CAD build for the part. Positions are in the model's coordinates, mm. A direction names the side the tool comes from. Round coordinates to 2 decimals unless told otherwise and drop trailing zeros. Loops run counter-clockwise (first coordinate to the right, second up) from the corner with the lowest first, then second, coordinate; pieces in that order, holes last. Notation, with made-up numbers: M 26,83 L 74,83 A20 ccw 74,122 Z; hole C -29.5,-24.5 d3. An arc over 180 degrees is marked long. Use a Markdown table: item, result. Add a question column.
(1) Band-saw the part on D-D, the plane y = -10.5. Write the cut outline in (x, z), and give its area (3 significant figures).
(2) Flat gauge pins, fed straight in: P1, Ø8, axis at x = 13.5, y = 5, coming from the +Z side; P2, Ø2, axis at y = -2, z = 27, coming from the +X side; P3, Ø1, axis at y = -4, z = 107, coming from the -X side; P4, Ø5, axis at x = 16.5, z = 101, coming from the -Y side. Where does each tip first touch, or does it go through?
(3) Which spindle directions (+Z, -Z, +X, -X, +Y, -Y) get a long thin tool onto all of the face, cutting with end or side? Do faces 1 (the face through (13.9, 0, 54)), 2 (the face through (-13.9, 0, 54)), 3 (the face through (0.42, -0.78, 135.95)). Say none if no direction does.
(4) Wall check: L1, parallel to Z at x = 7.5, y = 9; L2, parallel to X at y = -3.25, z = 33.5; L3, parallel to Y at x = -10.5, z = 129.5. Give the ranges that are in metal, low to high.
(5) Band-saw the part on A-A, the plane x = 0. Write the cut outline in (y, z), and give its area (3 significant figures).
(6) Band-saw the part on C-C, the plane z = 66.5. Write the cut outline in (x, y), and give its area (3 significant figures).
(7) Band-saw the part on B-B, the plane y = 0. Write the cut outline in (x, z).
from build123d import *

# Parameters (mm, degrees)
F0_W     = 27.8
F0_H     = 27.8
F1_DEPTH = 110
F2_R     = 6
F3_DEPTH = 20
F4_R     = 6
F5_DEPTH = 30


with BuildPart() as f1:
    # F0 (on Top) → F1 (new body)
    with BuildSketch(Plane.XY):
        Rectangle(F0_W, F0_H)
    extrude(amount=F1_DEPTH)

    # F2 (on face) → F3 (join)
    with BuildSketch(Plane.XY.offset(110)):
        Circle(F2_R)
    extrude(amount=F3_DEPTH)

    # F4 (on Right) → F5 (join, symmetric)
    with BuildSketch(Plane.YZ):
        with Locations((0, 130)):
            Circle(F4_R)
    extrude(amount=F5_DEPTH, both=True)


solid = f1.part
Return value:
| question | item | result |
|---|---|---|
| 1 | outline | M -13.9,0 L 13.9,0 L 13.9,110 L -13.9,110 Z |
| 1 | area | 3,060 mm^2 |
| 2 | P1 | z = 135.92 |
| 2 | P2 | x = 13.9 |
| 2 | P3 | x = -13.9 |
| 2 | P4 | through |
| 3 | face 1 | -Z, +X, +Y, -Y |
| 3 | face 2 | -Z, -X, +Y, -Y |
| 3 | face 3 | none |
| 4 | L1 | 0 to 110 |
| 4 | L2 | -13.9 to 13.9 |
| 4 | L3 | -5.98 to 5.98 |
| 5 | outline | M -13.9,0 L 13.9,0 L 13.9,110 L 6,110 L 6,130 A6 ccw -6,130 L -6,110 L -13.9,110 Z |
| 5 | area | 3,350 mm^2 |
| 6 | outline | M -13.9,-13.9 L 13.9,-13.9 L 13.9,13.9 L -13.9,13.9 Z |
| 6 | area | 773 mm^2 |
| 7 | outline | M -30,124 L -6,124 L -6,110 L -13.9,110 L -13.9,0 L 13.9,0 L 13.9,110 L 6,110 L 6,124 L 30,124 L 30,136 L -30,136 Z |
